```python
from build123d import *

# Parameters (mm, degrees)
SKETCH_1_R               = 28.4
EXTRUDE_1_DEPTH          = 6
SKETCH_2_R               = 12
EXTRUDE_2_DEPTH          = 20.4
CUT_EXTRUDE_1_DEPTH      = 46.047530454
CUT_EXTRUDE_1_DEPTH_BACK = 46.047530454
SKETCH_3_R               = 5
SKETCH_5_W               = 3.5
SKETCH_5_H               = 12
SKETCH_7_R               = 2.6
CUT_EXTRUDE_2_DEPTH      = 46.047530499
PATTERN_CIRCULAR_1_COUNT = 6


with BuildPart() as part:
    # ｽｹｯﾁ1 → ﾎﾞｽ - 押し出し1 (new body)
    with BuildSketch(Plane.XY):
        Circle(SKETCH_1_R)
    extrude(amount=EXTRUDE_1_DEPTH)

    # ｽｹｯﾁ2 → ﾎﾞｽ - 押し出し2 (add)
    with BuildSketch(Plane.XY):
        Circle(SKETCH_2_R)
    extrude(amount=-EXTRUDE_2_DEPTH)

    # ｽｹｯﾁ3 → ｶｯﾄ - 押し出し1 (cut, two sides: drawn at the far end of the back side and taken through both)
    with BuildSketch(Plane.XY.offset(-CUT_EXTRUDE_1_DEPTH_BACK)):
        Circle(SKETCH_3_R)
    extrude(amount=CUT_EXTRUDE_1_DEPTH + CUT_EXTRUDE_1_DEPTH_BACK, mode=Mode.SUBTRACT)

    # ｽｹｯﾁ5 → M6 すきま穴1 (revolve, cut)
    with BuildSketch(Plane(origin=(0, 0, -10.2), x_dir=(0, 0, 1), z_dir=(0, 1, 0))):
        with Locations((1.75, 6)):
            Rectangle(SKETCH_5_W, SKETCH_5_H)
    revolve(axis=Axis((-6.35, 0, -10.2), (1, 0, 0)), mode=Mode.SUBTRACT)

    # ｽｹｯﾁ7 → ｶｯﾄ - 押し出し2 (cut, symmetric)
    with BuildSketch(Plane.XY):
        with Locations((23.75, 0)):
            Circle(SKETCH_7_R)
    cut_extrude_2 = extrude(amount=CUT_EXTRUDE_2_DEPTH, both=True, mode=Mode.SUBTRACT)

    # 円形ﾊﾟﾀｰﾝ1: ｶｯﾄ - 押し出し2 ×6 about axis
    pattern_circular_1_axis = Axis((0, 0, 0), (0, 0, 1))
    for i in range(1, PATTERN_CIRCULAR_1_COUNT):
        add(cut_extrude_2.rotate(pattern_circular_1_axis, i * 360 / PATTERN_CIRCULAR_1_COUNT), mode=Mode.SUBTRACT)


solid = part.part
```
CAD build for the part. Positions are in the model's coordinates, mm. A direction names the side the tool comes from. Round coordinates to 2 decimals unless told otherwise and drop trailing zeros. Write each loop counter-clockwise with the first axis right and the second up, starting at its lowest first coordinate (ties: lowest second). Pieces come first, ordered by that corner, then holes.
Item 1: Band-saw the part on B-B on x = 0. Write the cut outline in (y, z).
Filled in:
outline: (-28.4, 0) - (-12, 0) - (-12, -20.4) - (-5, -20.4) - (-5, 6) - (-28.4, 6) - close; (5, -20.4) - (12, -20.4) - (12, 0) - (28.4, 0) - (28.4, 6) - (5, 6) - close
Item 2: Band-saw the part on D-D on x = 6. Write the cut outline in (y, z), then the cut area to 3 significant figures.
Filled in:
outline: (-27.76, 0) - (-10.39, 0) - (-10.39, -20.4) - (10.39, -20.4) - (10.39, 0) - (27.76, 0) - (27.76, 6) - (-27.76, 6) - close; hole circle Ø7 at (0, -10.2)
area: 719 mm2
Item 3: Drop flat-ended pins along their axis: pin 1 Ø10 at (x, z) = (12.5, 1.5) entering from +Y; pin 2 Ø6 at (x, y) = (-23.75, 0) entering from -Z; pin 3 Ø4 at (y, z) = (0, -10.2) entering from +X; pin 4 Ø3 at (x, y) = (11.88, -20.57) entering from -Z. Give the stop position or say it passes through.
Filled in:
pin 1: stops at y = 27.39
pin 2: stops at z = 0
pin 3: stops at x = -4.58
pin 4: passes through
Item 4: Drill centre lines: L1, parallel to Z at x = 10, y = 0; L2, parallel to Y at x = -13.5, z = 1.5; L3, parallel to Y at x = 0, z = -19. Where is each one in solid material? Low to high.
Filled in:
L1: z = -20.4 to -13.7, -6.7 to 6
L2: y = -24.99 to -22.6, -18.54 to 18.54, 22.6 to 24.99
L3: y = -12 to -5, 5 to 12
Item 5: Band-saw the part on A-A on y = 0. Write the cut outline in (x, z), then the cut area to 3 significant figures.
Filled in:
outline: (-28.4, 0) - (-26.35, 0) - (-26.35, 6) - (-28.4, 6) - close; (-21.15, 0) - (-12, 0) - (-12, -20.4) - (-5, -20.4) - (-5, 6) - (-21.15, 6) - close; (5, -20.4) - (12, -20.4) - (12, -13.7) - (5, -13.7) - close; (5, -6.7) - (12, -6.7) - (12, 0) - (21.15, 0) - (21.15, 6) - (5, 6) - close; (26.35, 0) - (28.4, 0) - (28.4, 6) - (26.35, 6) - close
area: 455 mm2
Item 6: Band-saw the part on C-C on y = 22. Write the cut outline in (x, z).
Filled in:
outline: (-17.96, 0) - (-14.05, 0) - (-14.05, 6) - (-17.96, 6) - close; (-9.7, 0) - (9.7, 0) - (9.7, 6) - (-9.7, 6) - close; (14.05, 0) - (17.96, 0) - (17.96, 6) - (14.05, 6) - close
Item 7: Mould opens along Z. For faces 3 (the cylindrical face through (10.68, -18.26, 3.04)), 4 (the cylindrical face through (7.844, 1.341, -6.967)), 5 (the flat face through (5.2, 0.2, -20.4)), 6 (the flat face through (6, 0, 6)) say: released by +Z, released by -Z, zero draft, split by the parting line, or undercut.
Filled in:
face 3: zero draft
face 4: undercut
face 5: released by -Z
face 6: released by +Z
Item 8: Tool access for faces 1 (the cylindrical face through (-12.439, -23.106, 3.042)), 2 (the cylindrical face through (-11.99, 0.53, -10.06)): list every direction of +Z, -Z, +X, -X, +Y, -Y with a clear straight run to the whole face (end or side of a thin tool).
Filled in:
face 1: +Z, -Z
face 2: -Z
